Source: CAD feature listing. Evaluate the final solid. Frame: model axes, mm. A direction names the side the tool comes from. Give positions to 0.01 mm unless a question says otherwise; leave off trailing zeros. Write each loop counter-clockwise with the first axis right and the second up, starting at its lowest first coordinate (ties: lowest second). Pieces come first, ordered by that corner, then holes. Notation, with made-up numbers: M 41,64 L 90,64 A19 ccw 90,78 Z; hole C -14,-27 d11. An arc over 180 degrees is marked long. Use CSV: the item, a comma, the result in double quotes. Start each with the question number.
from build123d import *

# Parameters (mm, degrees)
SKETCH1_W           = 133
SKETCH1_H           = 30
SKETCH1_R           = 1.75
SKETCH1_W_2         = 3
SKETCH1_H_2         = 10
BOSS_EXTRUDE1_DEPTH = 3


with BuildPart() as part:
    # Sketch1 → Boss-Extrude1 (new body)
    with BuildSketch(Plane.XY):
        with Locations((0, 2.5)):
            Rectangle(SKETCH1_W, SKETCH1_H)
        with Locations((-63, -7.5)):
            Circle(SKETCH1_R, mode=Mode.SUBTRACT)
        with Locations((63, -7.5)):
            Circle(SKETCH1_R, mode=Mode.SUBTRACT)
        with Locations((63, 6.5)):
            Rectangle(SKETCH1_W_2, SKETCH1_H_2, mode=Mode.SUBTRACT)
        with Locations((-63, 6.5)):
            Rectangle(SKETCH1_W_2, SKETCH1_H_2, mode=Mode.SUBTRACT)
    extrude(amount=BOSS_EXTRUDE1_DEPTH)


solid = part.part
Item 1: Set-up query: faces 4 (the flat face through (-1, 3, 3)), 5 (the flat face through (-61.5, 6, 1)). Return all of +Z, -Z, +X, -X, +Y, -Y with unobstructed straight access to the full face (end or side cutting, diameter ignored); none if empty.
Item 2: Section C-C (z = 1.3). Return the cut outline in (x, y).
Item 3: Section A-A (y = -7.5). Return the cut outline in (x, z), plus the area to 3 significant figures.
Item 4: Pull-direction query (X, two-part tool) for faces 1 (the cylindrical face through (64.669, -6.974, 1.479)), 2 (the flat face through (-66.5, 2, 1)), 3 (the flat face through (66.5, 2, 1)); classes: released by +X, released by -X, zero draft, split by the parting line, or undercut.
Item 5: Material intervals for probe 1 along X at (y, z) = (5.25, 1); probe 2 along Y at (x, z) = (63, 1.2); probe 3 along X at (y, z) = (-7.25, 2.8), sorted ascending.
Item 6: Section B-B (x = -63). Return the cut outline in (y, z).
Output values:
1,face 4,"+Z, +X, -X, +Y, -Y"
1,face 5,"+Z, -Z"
2,outline,"M -66.5,-12.5 L 66.5,-12.5 L 66.5,17.5 L -66.5,17.5 Z; hole C -63,-7.5 d3.5; hole M -64.5,1.5 L -61.5,1.5 L -61.5,11.5 L -64.5,11.5 Z; hole C 63,-7.5 d3.5; hole M 61.5,1.5 L 64.5,1.5 L 64.5,11.5 L 61.5,11.5 Z"
3,outline,"M -66.5,0 L -64.75,0 L -64.75,3 L -66.5,3 Z; M -61.25,0 L 61.25,0 L 61.25,3 L -61.25,3 Z; M 64.75,0 L 66.5,0 L 66.5,3 L 64.75,3 Z"
3,area,"378 mm2"
4,face 1,"undercut"
4,face 2,"released by -X"
4,face 3,"released by +X"
5,probe 1,"x = -66.5 to -64.5, -61.5 to 61.5, 64.5 to 66.5"
5,probe 2,"y = -12.5 to -9.25, -5.75 to 1.5, 11.5 to 17.5"
5,probe 3,"x = -66.5 to -64.73, -61.27 to 61.27, 64.73 to 66.5"
6,outline,"M -12.5,0 L -9.25,0 L -9.25,3 L -12.5,3 Z; M -5.75,0 L 1.5,0 L 1.5,3 L -5.75,3 Z; M 11.5,0 L 17.5,0 L 17.5,3 L 11.5,3 Z"
